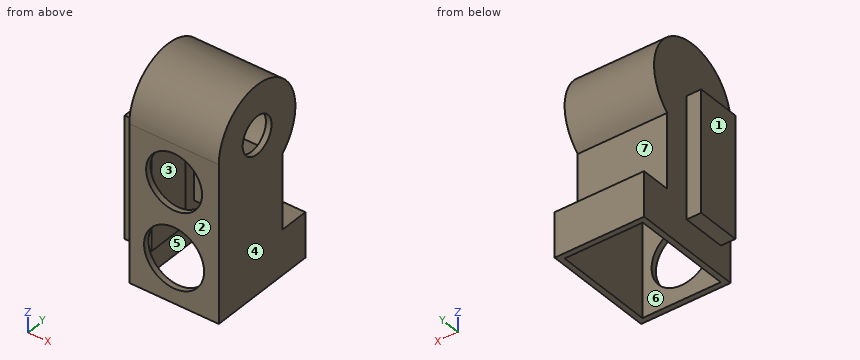
```python
from build123d import *

# Parameters (mm, degrees)
F1_DEPTH  = 12
F2_T      = -1.5
F3_R      = 5
F4_DEPTH  = 5
F5_R      = 7.5
F5_R_2    = 8.0533004945
F6_DEPTH  = 5
F10_START = -8.7
F9_W      = 11.8421060033
F9_H      = 32.5657902285
F10_DEPTH = 7.2


with BuildPart() as f1:
    # F0 (on Right) → F1 (new body, symmetric)
    with BuildSketch(Plane.YZ):
        with BuildLine():
            Line((0, 42), (0, 0))
            Line((0, 0), (30, 0))
            Line((30, 0), (30, 12))
            Line((30, 12), (22, 12))
            Line((22, 12), (22, 32))
            ThreePointArc((22, 32), (18.7650208971, 54.0830459736), (0, 42))
        make_face()
    extrude(amount=F1_DEPTH, both=True)

    # F2
    f2_openings = [f1.faces().sort_by_distance(p)[0] for p in [
        (0, 15, 0),
    ]]
    offset(amount=F2_T, openings=f2_openings, kind=Kind.INTERSECTION)

    # F3 (on face) → F4 (cut)
    with BuildSketch(Plane.YZ.offset(12)):
        with Locations((13.2727272727, 42)):
            Circle(F3_R)
    extrude(amount=-F4_DEPTH, mode=Mode.SUBTRACT)

    # F5 (on face) → F6 (cut)
    with BuildSketch(Plane.XZ):
        with Locations((0, 32)):
            Circle(F5_R)
        with Locations((0, 12)):
            Circle(F5_R_2)
    extrude(amount=-F6_DEPTH, mode=Mode.SUBTRACT)


with BuildPart() as f7_1:
    # F7: instance of F1
    add(f1.part.mirror(Plane(origin=(12, 12.8367440459, 24.8577602778), x_dir=(0, 1, 0), z_dir=(1, 0, 0))))


with BuildPart() as f1_1:
    add(f1.part)

    # F9 (on Right) → F10 (join)
    with BuildSketch(Plane.YZ.offset(F10_START)):
        with Locations((9.3256586697, 24.1282903589)):
            Rectangle(F9_W, F9_H)
    extrude(amount=-F10_DEPTH)


solid = f1_1.part
```
Read the model definition and answer for the solid it produces. Units are mm, in the model's axes. Face numbers are marked on the shaded views. A direction names the side the tool comes from. Round coordinates to 2 decimals unless told otherwise and drop trailing zeros. Loops run counter-clockwise (first coordinate to the right, second up) from the corner with the lowest first, then second, coordinate; pieces in that order, holes last. Notation, with made-up numbers: (27.25, 70) -> (32.25, 70) arc R28 cw to (32.25, 109) -> close; hole circle Ø9 at (27, -19). An arc over 180 degrees is marked (long way). One line per item, written item: value.
1) For the marked faces 4, 5, 6 and 7, determine the directions among +Z, -Z, +X, -X, +Y, -Y from which every point of the face is accessible in a straight line to the end or side of a thin tool.
Answer list:
face 4: +Z, -Z, +X, +Y, -Y
face 5: none
face 6: -Z
face 7: +X, -X, +Y
2) A cutting plane is placed at B-B (y = 25.75). Determine the outline of the cut face in (x, z), and give its area (3 significant figures).
Answer list:
outline: (-12, 0) -> (-10.5, 0) -> (-10.5, 10.5) -> (10.5, 10.5) -> (10.5, 0) -> (12, 0) -> (12, 12) -> (-12, 12) -> close; (-12, 37.47) -> (12, 37.47) -> (12, 46.53) -> (-12, 46.53) -> close
area: 285 mm²
3) A cutting plane is placed at D-D (y = 5.5). Determine the outline of the cut face in (x, z).
Answer list:
outline: (-15.9, 7.85) -> (-12, 7.85) -> (-12, 0) -> (-10.5, 0) -> (-10.5, 7.85) -> (-8.7, 7.85) -> (-8.7, 40.41) -> (-10.5, 40.41) -> (-10.5, 50.84) -> (10.5, 50.84) -> (10.5, 0) -> (12, 0) -> (12, 52.76) -> (-12, 52.76) -> (-12, 40.41) -> (-15.9, 40.41) -> close
4) Consider L1, parallel to Y at x = 1.25, z = 21.5; L2, parallel to X at y = 7.75, z = 11; L3, parallel to X at y = 20.75, z = 46.5. Determine where each line is inside the solid, lowest interval first. Write a range as [from, to].
Answer list:
L1: y = [0, 1.5], [20.5, 22]
L2: x = [-15.9, -8.7], [10.5, 12]
L3: x = [-12, -10.5], [10.5, 12]
5) Flat-ended cylindrical pins translate along their axes: P1, Ø13.5, axis at y = 18.5, z = 33.5, coming from the -X side; P2, Ø3, axis at x = 1.5, z = 30, coming from the -Y side; P3, Ø5, axis at x = -10, z = 27.5, coming from the +Y side; P4, Ø5, axis at x = 6.5, z = 30, coming from the +Y side. Find the tip coordinate at first contact, or state that the pin passes through.
Answer list:
P1: stops at x = -15.9
P2: stops at y = 20.5
P3: stops at y = 22
P4: stops at y = 22.54
6) A cutting plane is placed at C-C (z = 22.5). Determine the outline of the cut face in (x, y).
Answer list:
outline: (-15.9, 3.4) -> (-12, 3.4) -> (-12, 0) -> (12, 0) -> (12, 22) -> (-12, 22) -> (-12, 15.25) -> (-15.9, 15.25) -> close; hole (-10.5, 1.5) -> (10.5, 1.5) -> (10.5, 20.5) -> (-10.5, 20.5) -> (-10.5, 15.25) -> (-8.7, 15.25) -> (-8.7, 3.4) -> (-10.5, 3.4) -> close
7) A cutting plane is placed at A-A (x = 0). Determine the outline of the cut face in (y, z), and give its area (3 significant figures).
Answer list:
outline: (0, 0) -> (1.5, 0) -> (1.5, 3.95) -> (0, 3.95) -> close; (0, 20.05) -> (1.5, 20.05) -> (1.5, 24.5) -> (0, 24.5) -> close; (0, 39.5) -> (1.5, 39.5) -> (1.5, 42) arc R11.77 cw (long way) to (20.5, 32.71) -> (20.5, 10.5) -> (28.5, 10.5) -> (28.5, 0) -> (30, 0) -> (30, 12) -> (22, 12) -> (22, 32) arc R13.27 ccw (long way) to (0, 42) -> close
area: 152 mm²
8) The mould has two halves that part along Y. Classify the marked faces 1, 2 and 3: pulls with the +Y half, pulls with the -Y half, needs draft (parallel to the pull), parting line crosses it, or undercut.
Answer list:
face 1: needs draft
face 2: pulls with the -Y half
face 3: undercut
